Part model, mm, in its own coordinate system. Face numbers are marked on the shaded views. Round coordinates to 2 decimals unless told otherwise and drop trailing zeros. Write each loop counter-clockwise with the first axis right and the second up, starting at its lowest first coordinate (ties: lowest second). Pieces come first, ordered by that corner, then holes. Notation, with made-up numbers: M 57,9.5 L 69,9.5 A31 cw 69,46.5 Z; hole C 10,9.5 d10. An arc over 180 degrees is marked long. Answer as a JSON object with one key per item and string values. Group by question number.
1. Band-saw the part on D-D, the plane x = 168.5. Write the cut outline in (y, z).
2. Band-saw the part on A-A, the plane x = -21.5. Write the cut outline in (y, z).
3. Drill centre lines: line 1 (X direction, y = 50, z = -78); line 2 (Y direction, x = 18, z = 43); line 3 (Z direction, x = 18, y = 50). Where is each one in solid material? Low to high. Write a range as from..to.
4. Two-plate mould, pull along X, no slides. Class the marked faces 1 and 2: +X half, -X half, draft (parallel to the pull), parting line (faces both ways), or undercut.
5. Band-saw the part on C-C, the plane z = -11. Write the cut outline in (x, y).
6. Drop flat-ended pins along their axis: pin 1 (24 mm diameter, centred on y = 40.5, z = -4, fed in from +X); pin 2 (5 mm diameter, centred on x = -51.33, z = 23.8, fed in from -Y); pin 3 (24 mm diameter, centred on x = 19, y = 46, fed in from +Z). Give the stop position or say it passes through.
7. Band-saw the part on B-B, the plane z = 85.5. Write the cut outline in (x, y).
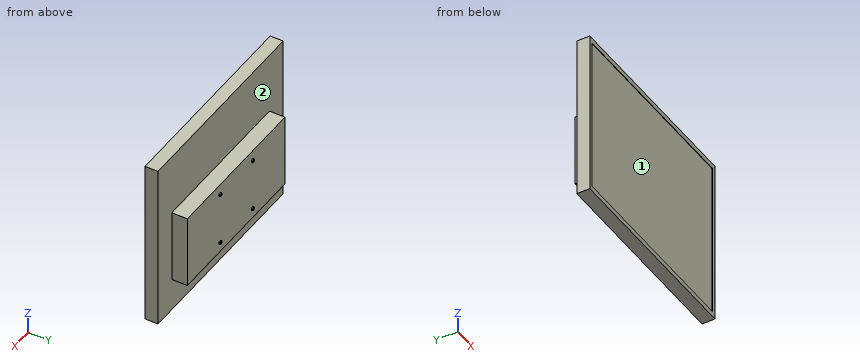
from build123d import *

# Parameters (mm, degrees)
SKETCH1_W           = 395
SKETCH1_H           = 325
BOSS_EXTRUDE1_DEPTH = 25
SKETCH2_W           = 380
SKETCH2_H           = 305
CUT_EXTRUDE1_DEPTH  = 0.8
SKETCH3_W           = 308
SKETCH3_H           = 142
SKETCH3_R           = 3.5
BOSS_EXTRUDE3_DEPTH = 30
SKETCH3_3_R         = 3.5
BOSS_EXTRUDE4_DEPTH = 32
SKETCH4_R           = 2
CUT_EXTRUDE2_DEPTH  = 10


with BuildPart() as part:
    # Sketch1 → Boss-Extrude1 (new body)
    with BuildSketch(Plane(origin=(0, 0, 0), x_dir=(1, 0, 0), z_dir=(0, 1, 0))):
        Rectangle(SKETCH1_W, SKETCH1_H)
    extrude(amount=BOSS_EXTRUDE1_DEPTH)

    # Sketch2 → Cut-Extrude1 (cut)
    with BuildSketch(Plane.XZ):
        Rectangle(SKETCH2_W, SKETCH2_H)
    extrude(amount=-CUT_EXTRUDE1_DEPTH, mode=Mode.SUBTRACT)

    # Sketch3 → Boss-Extrude3 (add)
    with BuildSketch(Plane(origin=(0, 25, 0), x_dir=(1, 0, 0), z_dir=(0, 1, 0))):
        with Locations((0, 27.2)):
            Rectangle(SKETCH3_W, SKETCH3_H)
        with Locations(Location((51.333333333, 78.2, 0), (0, 0, 270))):
            Circle(SKETCH3_R, mode=Mode.SUBTRACT)
        with Locations(Location((-51.333333333, 78.2, 0), (0, 0, 270))):
            Circle(SKETCH3_R, mode=Mode.SUBTRACT)
        with Locations(Location((51.333333333, -23.8, 0), (0, 0, 270))):
            Circle(SKETCH3_R, mode=Mode.SUBTRACT)
        with Locations(Location((-51.333333333, -23.8, 0), (0, 0, 270))):
            Circle(SKETCH3_R, mode=Mode.SUBTRACT)
    extrude(amount=BOSS_EXTRUDE3_DEPTH)

    # Sketch3_3 → Boss-Extrude4 (add)
    with BuildSketch(Plane(origin=(0, 25, 0), x_dir=(1, 0, 0), z_dir=(0, 1, 0))):
        with Locations(Location((-51.333333333, -23.8, 0), (0, 0, 270))):
            Circle(SKETCH3_3_R)
        with Locations(Location((51.333333333, -23.8, 0), (0, 0, 270))):
            Circle(SKETCH3_3_R)
        with Locations(Location((51.333333333, 78.2, 0), (0, 0, 270))):
            Circle(SKETCH3_3_R)
        with Locations(Location((-51.333333333, 78.2, 0), (0, 0, 270))):
            Circle(SKETCH3_3_R)
    extrude(amount=BOSS_EXTRUDE4_DEPTH)

    # Sketch4 → Cut-Extrude2 (cut)
    with BuildSketch(Plane(origin=(0, 57, 0), x_dir=(1, 0, 0), z_dir=(0, 1, 0))):
        with Locations(Location((-51.333333333, 78.2, 0), (0, 0, 270))):
            Circle(SKETCH4_R)
        with Locations(Location((51.333333333, 78.2, 0), (0, 0, 270))):
            Circle(SKETCH4_R)
        with Locations(Location((-51.333333333, -23.8, 0), (0, 0, 270))):
            Circle(SKETCH4_R)
        with Locations(Location((51.333333333, -23.8, 0), (0, 0, 270))):
            Circle(SKETCH4_R)
    extrude(amount=-CUT_EXTRUDE2_DEPTH, mode=Mode.SUBTRACT)


solid = part.part
Worked answers:
{
 "1": {"outline": "M 0,-162.5 L 25,-162.5 L 25,162.5 L 0,162.5 L 0,152.5 L 0.8,152.5 L 0.8,-152.5 L 0,-152.5 Z"},
 "2": {"outline": "M 0,-162.5 L 25,-162.5 L 25,-98.2 L 55,-98.2 L 55,43.8 L 25,43.8 L 25,162.5 L 0,162.5 L 0,152.5 L 0.8,152.5 L 0.8,-152.5 L 0,-152.5 Z"},
 "3": {"line 1": "x = -154..-53.32, -49.34..49.34, 53.32..154", "line 2": "y = 0.8..55", "line 3": "z = -98.2..43.8"},
 "4": {"face 1": "undercut", "face 2": "draft"},
 "5": {"outline": "M -197.5,0 L -190,0 L -190,0.8 L 190,0.8 L 190,0 L 197.5,0 L 197.5,25 L 154,25 L 154,55 L -154,55 L -154,25 L -197.5,25 Z"},
 "6": {"pin 1": "stops at x = 154", "pin 2": "stops at y = 0.8", "pin 3": "stops at z = 43.8"},
 "7": {"outline": "M -197.5,0 L -190,0 L -190,0.8 L 190,0.8 L 190,0 L 197.5,0 L 197.5,25 L -197.5,25 Z"}
}
